CAD build for the part. Positions are in the model's coordinates, mm. A direction names the side the tool comes from. Coordinates: 2 decimals unless noted, no trailing zeros. Loops run counter-clockwise (first coordinate to the right, second up) from the corner with the lowest first, then second, coordinate; pieces in that order, holes last. Notation, with made-up numbers: (8, -30.75) -> (58, -30.75) arc R21 cw to (58, 4.25) -> close; hole circle Ø10 at (39, -10.75). An arc over 180 degrees is marked (long way). Write item = value, one per line. Start each with the question number.
(1) Flat gauge pins, fed straight in: P1, Ø10.5, axis at x = 5.4, z = -2.79, coming from the -Y side; P2, Ø4, axis at x = -27.94, y = 0, coming from the -Z side; P3, Ø6.5, axis at y = 0, z = -13, coming from the +X side; P4, Ø6.5, axis at y = 2, z = -18.5, coming from the -X side. Where does each tip first touch, or does it go through?
(2) Drill centre lines: line 1 (X direction, y = 4.5, z = -2.5); line 2 (X direction, y = 2.5, z = -19); line 3 (Z direction, x = -6.5, y = 4.5). Where is each one in solid material? Low to high. Write a range as from..to.
(3) Band-saw the part on B-B (z = 33.5). Write the cut outline in (x, y), and give its area (3 significant figures).
(4) Tool access for faces 1 (the face through (0, 0, 0)), 2 (the face through (12, -0.089, -28.486)), 3 (the face through (9.544, 0.553, -15.573)): list every direction of +Z, -Z, +X, -X, +Y, -Y with a clear straight run to the whole face (end or side of a thin tool).
(5) Band-saw the part on A-A (x = 0). Write the cut outline in (y, z) (3 decimals), and give its area (3 significant figures).
(6) Pull direction Z, two halves, no side cores. Call faces 4 (the face through (-6.414, 0, -13)), 5 (the face through (-26.29, 0.07, 29.91)), 6 (the face through (26, -2, 37.338)), 7 (the face through (6.414, 3, -13)): +Z half, -Z half, draft (parallel to the pull), parting line (faces both ways), or undercut.
(7) Band-saw the part on D-D (x = -27.94). Write the cut outline in (y, z), and give its area (3 significant figures).
```python
from build123d import *

# Parameters (mm, degrees)
F0_W     = 12.827
F0_H     = 26.162
F1_DEPTH = 6.35
F3_D     = 5.1054
F3_DEPTH = 26.6075
F5_D     = 3.3
F6_R     = 3.302
F7_DEPTH = 12.701
F8_R     = 2.54
F9_R     = 7.62
F10_R    = 7.62


# Not quite as in the source:
# - a pattern or mirror of a feature is missing from the dataset's text; its kind, count and spacing are read off the source's solid


with BuildPart() as f1:
    # F0 (on Front) → F1 (new body, symmetric)
    with BuildSketch(Plane.XZ):
        with BuildLine():
            Line((-12.7635, -29.21), (12.7635, -29.21))
            Line((12.7635, -29.21), (12.7635, 0))
            Line((12.7635, 0), (33.02, 27.94))
            Line((33.02, 27.94), (33.02, 37.338))
            Line((33.02, 37.338), (22.2119333017, 37.338))
            ThreePointArc((22.2119333017, 37.338), (0, 15.875), (-22.2119333017, 37.338))
            Line((-22.2119333017, 37.338), (-33.02, 37.338))
            Line((-33.02, 37.338), (-33.02, 27.94))
            Line((-33.02, 27.94), (-12.7635, 0))
            Line((-12.7635, 0), (-12.7635, -29.21))
        make_face()
        with Locations((0, -13.081)):
            Rectangle(F0_W, F0_H, mode=Mode.SUBTRACT)
    extrude(amount=F1_DEPTH, both=True)

    # F3 (through all, one way)
    with BuildSketch(Plane(origin=(6.4135, 0, 0), x_dir=(0, -1, 0), z_dir=(-1, 0, 0))):
        with Locations((0, -13.081)):
            Circle(F3_D / 2)
    extrude(amount=-F3_DEPTH, mode=Mode.SUBTRACT)

    # F5 (through all)
    with Locations(Plane.XY.offset(37.338)):
        with Locations((-27.94, 0)):
            f5 = Hole(F5_D / 2)

    # F5_copies: F5 across plane
    add(f5.mirror(Plane(origin=(6e-06, 0, 0), x_dir=(0, 0, 1), z_dir=(1, 0, 0))), mode=Mode.SUBTRACT)

    # F6 (on face) → F7 (cut, through all)
    with BuildSketch(Plane.XZ.offset(6.35)):
        with Locations((-5.3975, -2.794)):
            Circle(F6_R)
        with Locations((-5.3975, -23.368)):
            Circle(F6_R)
        with Locations((5.3975, -2.794)):
            Circle(F6_R)
        with Locations((5.3975, -23.368)):
            Circle(F6_R)
    extrude(amount=-F7_DEPTH, mode=Mode.SUBTRACT)

    # F8
    f8_edges = [f1.edges().sort_by_distance(p)[0] for p in [
        (12.7635, 0, -29.21),
        (-12.7635, 0, -29.21),
    ]]
    fillet(f8_edges, radius=F8_R)

    # F9
    f9_edges = [f1.edges().sort_by_distance(p)[0] for p in [
        (12.7635, 0, 0),
        (-12.7635, 0, 0),
    ]]
    fillet(f9_edges, radius=F9_R)

    # F10
    f10_edges = [f1.edges().sort_by_distance(p)[0] for p in [
        (33.02, 0, 27.94),
        (-33.02, 0, 27.94),
    ]]
    fillet(f10_edges, radius=F10_R)


solid = f1.part
```
Findings below:
q1.P1 = -6.35
q1.P2 = 18.17
q1.P3 = 12.76
q1.P4 = -12.76
q2.line_1 = -12.76..-8.69, 8.69..12.76
q2.line_2 = -12.76..-6.41, 6.41..12.76
q2.line_3 = -29.21..-26.48, -20.26..-5.91, 0.32..16.85
q3.outline = (-33.02, -6.35) -> (-21.74, -6.35) -> (-21.74, 6.35) -> (-33.02, 6.35) -> close; (21.74, -6.35) -> (33.02, -6.35) -> (33.02, 6.35) -> (21.74, 6.35) -> close; hole circle Ø3.3 at (-27.94, 0); hole circle Ø3.3 at (27.94, 0)
q3.area = 269 mm²
q4.face_1 = +Y, -Y
q4.face_2 = -Z, +X, +Y, -Y
q4.face_3 = +X
q5.outline = (-6.35, -29.21) -> (6.35, -29.21) -> (6.35, -26.162) -> (-6.35, -26.162) -> close; (-6.35, 0) -> (6.35, 0) -> (6.35, 15.875) -> (-6.35, 15.875) -> close
q5.area = 240 mm²
q6.face_4 = undercut
q6.face_5 = draft
q6.face_6 = +Z half
q6.face_7 = undercut
q7.outline = (-6.35, 20.93) -> (-1.65, 20.93) -> (-1.65, 37.34) -> (-6.35, 37.34) -> close; (1.65, 20.93) -> (6.35, 20.93) -> (6.35, 37.34) -> (1.65, 37.34) -> close
q7.area = 154 mm²
